from build123d import *

# Parameters (mm, degrees)
BOSS_EXTRUDE1_DEPTH   = 40
BODY_MOVE_COPY1_ANGLE = 20
BOSS_EXTRUDE2_DEPTH   = 2
BOSS_EXTRUDE3_DEPTH   = 12
SKETCH4_R             = 2.5
CUT_EXTRUDE2_DEPTH    = 8
FILLET1_R             = 2
SKETCH10_W            = 4.9
SKETCH10_H            = 3
SKETCH10_W_2          = 5.1
SKETCH10_W_3          = 5
CUT_EXTRUDE4_DEPTH    = 2
FILLET2_R             = 0.5


with BuildPart() as part:
    # Sketch2 → Boss-Extrude1 (new body)
    with BuildSketch(Plane.XY):
        Polygon((90, 0), (102, 0), (102, 2), (92, 25), (90, 25), align=None)
    extrude(amount=BOSS_EXTRUDE1_DEPTH)


with BuildPart() as part_1:
    # Body-Move/Copy1: moved
    add(part.part.rotate(Axis((95, 0, 20), (0, -1, 0)), BODY_MOVE_COPY1_ANGLE))


with BuildPart() as part_2:
    # Body-Move/Copy2: moved
    add(part_1.part.moved(Location((-4, 0, -25))))

    # Sketch1 → Boss-Extrude2 (add)
    with BuildSketch(Plane(origin=(0, 0, 0), x_dir=(1, 0, 0), z_dir=(0, 1, 0))):
        Polygon((0, 49), (0, 0), (73, 0), (84, -12), (87, 0), (87, 49), align=None)
    extrude(amount=BOSS_EXTRUDE2_DEPTH)

    # Sketch1<4> → Boss-Extrude3 (add)
    with BuildSketch(Plane(origin=(0, 0, 0), x_dir=(1, 0, 0), z_dir=(0, 1, 0))):
        Polygon((8, 43), (8, 46), (39.9, 46), (39.9, 43), (44.9, 43), (44.9, 46), (79, 46), (79, 43), (83.9, 43), (83.9, 6), (79, 6), (79, 3), (44.9, 3), (44.9, 6), (39.9, 6), (39.9, 3), (8, 3), (8, 6), (2.9, 6), (2.9, 13), (0, 13), (0, 0), (73, 0), (87, 0), (87, 49), (0, 49), (0, 36), (2.9, 36), (2.9, 43), align=None)
    extrude(amount=BOSS_EXTRUDE3_DEPTH)

    # Sketch4 → Cut-Extrude2 (cut)
    with BuildSketch(Plane(origin=(72.447790922, 33.520577724, 26.368839434), x_dir=(0.30020671045987535, 0.09758957417323016, -0.948868908757974), z_dir=(0.8617639646050662, 0.3987261114144503, 0.31365643207890637))):
        with Locations(Location((42.044187921, -18.952687866, 0), (0, 0, 92.148700458))):
            Circle(SKETCH4_R)
        with Locations(Location((40.341555526, -34.861837527, 0), (0, 0, 92.148700458))):
            Circle(SKETCH4_R)
    extrude(amount=-CUT_EXTRUDE2_DEPTH, mode=Mode.SUBTRACT)

    # Fillet1
    fillet1_edges = [part_2.edges().sort_by_distance(p)[0] for p in [
        (80.40082665, 25, 12.425771842),
        (94.081632383, 25, -25.161932989),
    ]]
    fillet(fillet1_edges, radius=FILLET1_R)

    # Sketch10 → Cut-Extrude4 (cut)
    with BuildSketch(Plane(origin=(0, 12, 0), x_dir=(1, 0, 0), z_dir=(0, 1, 0))):
        with Locations((81.45, 4.5)):
            Rectangle(SKETCH10_W, SKETCH10_H)
        with Locations((42.45, 4.5)):
            Rectangle(SKETCH10_W_2, SKETCH10_H)
        with Locations((42.4, 44.5)):
            Rectangle(SKETCH10_W_3, SKETCH10_H)
        with Locations((81.45, 44.5)):
            Rectangle(SKETCH10_W, SKETCH10_H)
        with Locations((5.45, 44.5)):
            Rectangle(SKETCH10_W_2, SKETCH10_H)
        with Locations((5.45, 4.5)):
            Rectangle(SKETCH10_W_2, SKETCH10_H)
    extrude(amount=-CUT_EXTRUDE4_DEPTH, mode=Mode.SUBTRACT)

    # Fillet2
    fillet2_edges = [part_2.edges().sort_by_distance(p)[0] for p in [
        (86.301536896, 25, -6.710100717),
        (79.46113403, 11.5, 12.083751699),
        (93.141939763, 11.5, -25.503953132),
        (79.661484791, 24.414213562, 11.533292506),
        (92.941589001, 24.414213562, -24.95349394),
        (87, 6, -49),
        (0, 6, -49),
        (0, 6, 0),
        (2.9, 12, -41),
        (43.4, 12, -46),
        (83.9, 12, -24.5),
        (2.9, 12, -8),
        (43.4, 12, -3),
    ]]
    fillet(fillet2_edges, radius=FILLET2_R)


solid = part_2.part
Read the model definition and answer for the solid it produces. Units are mm, in the model's axes. A direction names the side the tool comes from. Coordinates: 2 decimals unless noted, no trailing zeros. Order: outer loops, then holes, each group sorted by start corner. A loop starts at its lowest first (then second) coordinate and runs counter-clockwise, first axis right, second up. Notation, with made-up numbers: (35, -2) -> (61, -2) arc R29 ccw to (61, 30) -> close; hole circle Ø11 at (85.5, -20.75). An arc over 180 degrees is marked (long way). Answer as a JSON object with one key per item and string values.
1) Each of these flat-tipped pins is pushed along its axis until it touches: pin 1 (13 mm diameter, centred on x = 46, z = -19, fed in from +Y); pin 2 (10 mm diameter, centred on y = 10, z = 7, fed in from +X); pin 3 (5 mm diameter, centred on y = 8.5, z = -24.5, fed in from -X); pin 4 (5 mm diameter, centred on x = 51.5, y = 16, fed in from -Z). Where does it stop, or does it pass through?
Model answer:
{"pin 1": "stops at y = 2", "pin 2": "stops at x = 93.32", "pin 3": "stops at x = 83.9", "pin 4": "passes through"}
2) A cutting plane is placed at A-A, the plane z = -38.5. Determine the outline of the cut face in (x, y), plus the area to 3 significant figures.
Model answer:
{"outline": "(0, 0) -> (87, 0) -> (87, 12) -> (84.4, 12) arc R0.5 ccw to (83.9, 11.5) -> (83.9, 2) -> (2.9, 2) -> (2.9, 11.5) arc R0.5 ccw to (2.4, 12) -> (0, 12) -> close", "area": "234 mm²"}
3) A cutting plane is placed at D-D, the plane x = 77.5. Determine the outline of the cut face in (y, z).
Model answer:
{"outline": "(0, -49) -> (12, -49) -> (12, -46.5) arc R0.5 ccw to (11.5, -46) -> (2, -46) -> (2, -3) -> (11.5, -3) arc R0.5 ccw to (12, -2.5) -> (12, 0) -> (2, 0) -> (2, 4.91) -> (0, 4.91) -> close"}
4) The mould has two halves that part along Y. Classify faces 4 (the face through (91.926, 2.442, -13.145)), 5 (the face through (86.35, 24.85, -6.42)), 6 (the face through (0, 1, -25)): released by +Y, released by -Y, zero draft, split by the parting line, or undercut.
Model answer:
{"face 4": "undercut", "face 5": "released by +Y", "face 6": "zero draft"}
5) A tool of negligible diameter and unlimited length cuts with its end or side. For faces 1 (the face through (94.267, 24.399, -24.488)), 2 (the face through (79, 6, -45)), 3 (the face through (87, 6, -28)), from which of +Z, -Z, +X, -X, +Y, -Y can it reach the whole face along a straight path? Write none if from no direction.
Model answer:
{"face 1": "-Z, +X, +Y", "face 2": "+Y", "face 3": "-Z, +Y, -Y"}
6) A cutting plane is placed at B-B, the plane x = 32. Determine the outline of the cut face in (y, z).
Model answer:
{"outline": "(0, -49) -> (12, -49) -> (12, -46.5) arc R0.5 ccw to (11.5, -46) -> (2, -46) -> (2, -3) -> (11.5, -3) arc R0.5 ccw to (12, -2.5) -> (12, 0) -> (0, 0) -> close"}
7) A cutting plane is placed at C-C, the plane y = 14.5. Determine the outline of the cut face in (x, z).
Model answer:
{"outline": "(79.63, 11.61) -> (92.97, -25.03) arc R0.5 ccw to (93.61, -25.33) -> (99.31, -23.26) -> (85.63, 14.33) -> (79.93, 12.25) arc R0.5 ccw to start"}
8) Consider line 1 along Z through (x, y) = (79.5, 9.25); line 2 along Y through (x, z) = (63, -9.5); line 3 along Z through (x, y) = (70, 5). Determine where each line is inside the solid, lowest interval first. Write a range as from..to.
Model answer:
{"line 1": "z = -49..-43, -6..0", "line 2": "y = 0..2", "line 3": "z = -49..-46, -3..0"}
